Could you check a few things on this model? Use its own coordinates, in mm. Face numbers are marked on the shaded views. Give positions to 0.01 mm unless a question says otherwise; leave off trailing zeros. Loops run counter-clockwise (first coordinate to the right, second up) from the corner with the lowest first, then second, coordinate; pieces in that order, holes last. Notation, with made-up numbers: M 0.25,19.5 L 59.25,19.5 A27 ccw 59.25,39.5 Z; hole C 73,20 d3. An arc over 180 degrees is marked long. Answer in a Markdown table with one row per item. Add a question column.
1. If we section it at D-D on z = 25: List the corners of the cut face in (x, y) for me, then the cut area to 3 significant figures.
2. If we section it at C-C on x = 0: List the corners of the cut face in (y, z) for me, then the cut area to 3 significant figures.
3. I'm going to push flat-ended pins straight in: pin 1 Ø10 at (x, z) = (9.5, 16) entering from -Y; pin 2 Ø1 at (x, z) = (-10.5, 25.5) entering from +Y; pin 3 Ø1 at (x, y) = (11, 10.5) entering from +Z. Where does each tip first touch, or does it pass through?
4. If we section it at A-A on y = 0: List the corners of the cut face in (x, z) for me, then the cut area to 3 significant figures.
5. If we section it at B-B on z = 9.75: List the corners of the cut face in (x, y) for me, then the cut area to 3 significant figures.
6. Thinking about a two-plate mould opening in Y: for the marked faces 1, 2 and 3, which applies, released by +Y, released by -Y, zero draft, split by the parting line, or undercut?
7. I need wall thicknesses on line 1 along X through (y, z) = (18.25, 5); line 2 along Y through (x, z) = (-0.25, 19.25); line 3 along Y through (x, z) = (12.75, 24). Which ranges of each line are inside material? Lowest first, please. Write a range as from..to.
```python
from build123d import *

# Parameters (mm, degrees)
BOSS_EXTRUDE1_DEPTH = 30
CUT_EXTRUDE2_START  = -20
SKETCH4_R           = 1.6
CUT_EXTRUDE2_DEPTH  = 20
SKETCH2_R           = 11.25
CUT_EXTRUDE3_DEPTH  = 30
SKETCH5_R           = 1.6
CUT_EXTRUDE4_DEPTH  = 9
FILLET1_R           = 0.5


with BuildPart() as part:
    # Sketch1 → Boss-Extrude1 (new body)
    with BuildSketch(Plane.XY):
        with BuildLine():
            Line((-15, 23.151243445), (-15, -13.228756555))
            ThreePointArc((-15, -13.228756555), (0, -20), (15, -13.228756555))
            Line((15, -13.228756555), (15, 23.151243445))
            Line((15, 23.151243445), (-15, 23.151243445))
        make_face()
    extrude(amount=BOSS_EXTRUDE1_DEPTH)

    # Sketch4 → Cut-Extrude2 (cut)
    with BuildSketch(Plane(origin=(0, 0, 0), x_dir=(-1, 0, 0), z_dir=(0, 0, -1)).offset(CUT_EXTRUDE2_START)):
        with Locations((-11.313708499, 11.313708499)):
            Circle(SKETCH4_R)
        with Locations((0, 16)):
            Circle(SKETCH4_R)
        with Locations((11.313708499, 11.313708499)):
            Circle(SKETCH4_R)
    cut_extrude2 = extrude(amount=-CUT_EXTRUDE2_DEPTH, mode=Mode.SUBTRACT)

    # Mirror1: Cut-Extrude2 across plane
    add(cut_extrude2.mirror(Plane.ZX), mode=Mode.SUBTRACT)

    # Sketch2 → Cut-Extrude3 (cut)
    with BuildSketch(Plane(origin=(0, 0, 0), x_dir=(-1, 0, 0), z_dir=(0, 0, -1))):
        Circle(SKETCH2_R)
    extrude(amount=-CUT_EXTRUDE3_DEPTH, mode=Mode.SUBTRACT)

    # Sketch5 → Cut-Extrude4 (cut)
    with BuildSketch(Plane(origin=(0, 23.151243445, 0), x_dir=(1, 0, 0), z_dir=(0, 1, 0))):
        with Locations(Location((10, -25, 0), (0, 0, 90))):
            Circle(SKETCH5_R)
        with Locations(Location((-10, -25, 0), (0, 0, 270))):
            Circle(SKETCH5_R)
        with Locations(Location((10, -5, 0), (0, 0, 270))):
            Circle(SKETCH5_R)
        with Locations(Location((-10, -5, 0), (0, 0, 90))):
            Circle(SKETCH5_R)
    extrude(amount=-CUT_EXTRUDE4_DEPTH, mode=Mode.SUBTRACT)

    # Fillet1
    fillet1_edges = [part.edges().sort_by_distance(p)[0] for p in [
        (15, 23.151243445, 15),
        (15, -13.228756555, 15),
        (-15, -13.228756555, 15),
        (-15, 23.151243445, 15),
    ]]
    fillet(fillet1_edges, radius=FILLET1_R)


solid = part.part
```
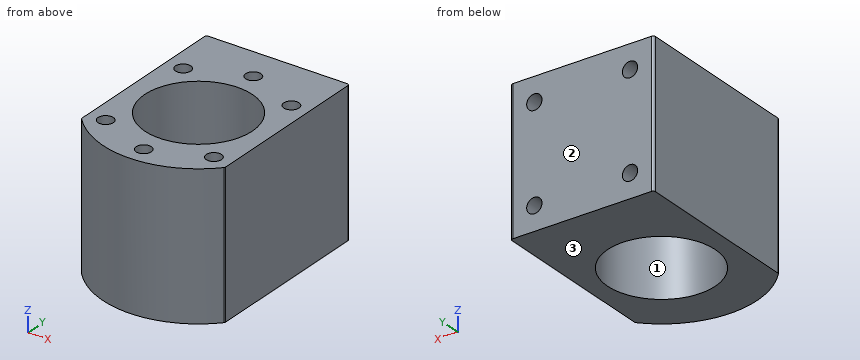
Results:
| question | item | result |
|---|---|---|
| 1 | outline | M -15,-13.04 A0.5 ccw -14.87,-13.37 A20 ccw 14.87,-13.37 A0.5 ccw 15,-13.04 L 15,22.65 A0.5 ccw 14.5,23.15 L 11.6,23.15 L 11.6,14.15 L 8.4,14.15 L 8.4,23.15 L -8.4,23.15 L -8.4,14.15 L -11.6,14.15 L -11.6,23.15 L -14.5,23.15 A0.5 ccw -15,22.65 Z; hole C -11.31,-11.31 d3.2; hole C -11.31,11.31 d3.2; hole C 0,0 d22.5; hole C 0,-16 d3.2; hole C 0,16 d3.2; hole C 11.31,-11.31 d3.2; hole C 11.31,11.31 d3.2 |
| 1 | area | 729 mm2 |
| 2 | outline | M -20,0 L -11.25,0 L -11.25,30 L -14.4,30 L -14.4,20 L -17.6,20 L -17.6,30 L -20,30 Z; M 11.25,0 L 23.15,0 L 23.15,30 L 17.6,30 L 17.6,20 L 14.4,20 L 14.4,30 L 11.25,30 Z |
| 2 | area | 556 mm2 |
| 3 | pin 1 | y = -19.49 |
| 3 | pin 2 | y = 14.15 |
| 3 | pin 3 | z = 20 |
| 4 | outline | M -15,0 L -11.25,0 L -11.25,30 L -15,30 Z; M 11.25,0 L 15,0 L 15,30 L 11.25,30 Z |
| 4 | area | 225 mm2 |
| 5 | outline | M -15,-13.04 A0.5 ccw -14.87,-13.37 A20 ccw 14.87,-13.37 A0.5 ccw 15,-13.04 L 15,22.65 A0.5 ccw 14.5,23.15 L -14.5,23.15 A0.5 ccw -15,22.65 Z; hole C 0,0 d22.5 |
| 5 | area | 834 mm2 |
| 6 | face 1 | undercut |
| 6 | face 2 | released by +Y |
| 6 | face 3 | zero draft |
| 7 | line 1 | -15..-11.6, -8.4..8.4, 11.6..15 |
| 7 | line 2 | -20..-11.25, 11.25..23.15 |
| 7 | line 3 | -15.41..-12.02, -10.61..10.61, 12.02..23.15 |
